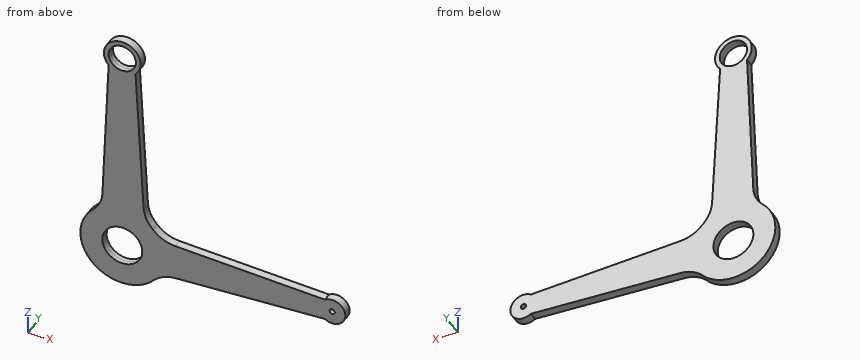
```python
from build123d import *

# Parameters (mm, degrees)
F0_R        = 19.0457812865
F0_R_2      = 13
F0_R_3      = 2.5
F1_DEPTH    = 4
F2_R        = 30
F3_R        = 30
F4_T1_DEPTH = 8
F5_R        = 30


# Not quite as in the source:
# - a fillet or chamfer that OpenCascade refuses, or shapes differently, is made with other operations: its cross-section is extruded or revolved along the edge and cut away or added


with BuildPart() as f1:
    # F0 (on Front) → F1 (new body, symmetric)
    with BuildSketch(Plane.XZ):
        with BuildLine():
            ThreePointArc((-19.5365896508, 34.9044648264), (0.8487956626, 39.99099331), (21, 34.0440890611))
            Line((21, 34.0440890611), (12.6265428967, 187.8830525924))
            ThreePointArc((12.6265428967, 187.8830525924), (-0.2904480488, 182.5024104537), (-13.0217419566, 188.3087966224))
            Line((-13.0217419566, 188.3087966224), (-19.5365896508, 34.9044648264))
        make_face()
        with BuildLine():
            ThreePointArc((35.8133699363, 17.8157945038), (38.939278354, 9.1505519655), (40, 0))
            ThreePointArc((40, 0), (38.9395050251, -9.1495873352), (35.8142525798, -17.8140201007))
            Line((35.8142525798, -17.8140201007), (192.9463185859, -10.3196694961))
            ThreePointArc((192.9463185859, -10.3196694961), (187.5000024995, 0.0079048318), (192.9593762653, 10.3285825468))
            Line((192.9593762653, 10.3285825468), (35.8133699363, 17.8157945038))
        make_face()
        with BuildLine():
            ThreePointArc((35.8142525798, -17.8140201007), (38.9395050251, -9.1495873352), (40, 0))
            ThreePointArc((40, 0), (38.939278354, 9.1505519655), (35.8133699363, 17.8157945038))
            ThreePointArc((35.8133699363, 17.8157945038), (29.542835628, 26.9670328931), (21, 34.0440890611))
            ThreePointArc((21, 34.0440890611), (0.8487956626, 39.99099331), (-19.5365896508, 34.9044648264))
            ThreePointArc((-19.5365896508, 34.9044648264), (-27.5871390481, -28.9646294494), (35.8142525798, -17.8140201007))
        make_face()
        Circle(F0_R, mode=Mode.SUBTRACT)
        with BuildLine():
            ThreePointArc((-13.0217419566, 188.3087966224), (-0.2904480488, 182.5024104537), (12.6265428967, 187.8830525924))
            ThreePointArc((12.6265428967, 187.8830525924), (16.2359862757, 193.4698583741), (17.5, 200))
            ThreePointArc((17.5, 200), (-6.2597729895, 216.3421308929), (-13.0217419566, 188.3087966224))
        make_face()
        with Locations((0, 200)):
            Circle(F0_R_2, mode=Mode.SUBTRACT)
        with BuildLine():
            ThreePointArc((212.5, 0), (205.841327046, 11.0511944306), (192.9593762653, 10.3285825468))
            ThreePointArc((192.9593762653, 10.3285825468), (187.5000024995, 0.0079048318), (192.9463185859, -10.3196694961))
            ThreePointArc((192.9463185859, -10.3196694961), (205.8343372513, -11.0548861974), (212.5, 0))
        make_face()
        with Locations((200, 0)):
            Circle(F0_R_3, mode=Mode.SUBTRACT)
    extrude(amount=F1_DEPTH, both=True)

    # F2
    f2_edges = [f1.edges().sort_by_distance(p)[0] for p in [
        (35.81337, 0, 17.815795),
    ]]
    fillet(f2_edges, radius=F2_R)

    # F3
    f3_edges = [f1.edges().sort_by_distance(p)[0] for p in [
        (21, 0, 34.044089),
    ]]
    fillet(f3_edges, radius=F3_R)

    # F4: fillet of radius 30 on 1 edges, made by hand

    # F4_s2 → F4_t1 (join)
    with BuildSketch(Plane.XZ.offset(-4)):
        with BuildLine():
            ThreePointArc((-18.9466482885, 48.7957428331), (-21.5235892515, 37.8433937284), (-27.954075006, 28.6106569403))
            ThreePointArc((-27.954075006, 28.6106569403), (-23.9529499606, 32.0352335435), (-19.5365896508, 34.9044648264))
            Line((-19.5365896508, 34.9044648264), (-18.9466482885, 48.7957428331))
        make_face()
    extrude(amount=F4_T1_DEPTH)

    # F5
    f5_edges = [f1.edges().sort_by_distance(p)[0] for p in [
        (35.814253, 0, -17.81402),
    ]]
    fillet(f5_edges, radius=F5_R)


solid = f1.part
```
Part model, mm, in its own coordinate system. Give positions to 0.01 mm unless a question says otherwise; leave off trailing zeros. Order: outer loops, then holes, each group sorted by start corner. A loop starts at its lowest first (then second) coordinate and runs counter-clockwise, first axis right, second up. Notation, with made-up numbers: (-13.5, -12.5) - (23.5, -12.5) arc R27 cw to (23.5, 11.5) - close; hole circle Ø11 at (18, 84). An arc over 180 degrees is marked (long way). Use one line per item in the form item = value.
Item 1: Slice it at A-A on y = 2.75. Give the cut face in (x, z).
Solution:
outline = (-27.95, 28.61) arc R40 ccw (long way) to (29.6, -26.91) arc R30 cw to (50.37, -17.12) - (192.95, -10.32) arc R12.5 ccw (long way) to (192.96, 10.33) - (50.37, 17.12) arc R30 cw to (29.6, 26.91) arc R40 ccw to (28.71, 27.85) arc R30 cw to (20.29, 47.11) - (12.63, 187.88) arc R17.5 ccw (long way) to (-13.02, 188.31) - (-18.95, 48.8) arc R30 cw to start; hole circle Ø38.09 at (0, 0); hole circle Ø26 at (0, 200); hole circle Ø5 at (200, 0)
Item 2: Slice it at C-C on z = 200. Give the cut face in (x, y).
Solution:
outline = (-17.5, -4) - (-13, -4) - (-13, 4) - (-17.5, 4) - close; (13, -4) - (17.5, -4) - (17.5, 4) - (13, 4) - close
Item 3: Slice it at B-B on x = 0. Give the cut face in (y, z), and give its area (3 significant figures).
Solution:
outline = (-4, -40) - (4, -40) - (4, -19.05) - (-4, -19.05) - close; (-4, 19.05) - (4, 19.05) - (4, 187) - (-4, 187) - close; (-4, 213) - (4, 213) - (4, 217.5) - (-4, 217.5) - close
area = 1,550 mm2
Item 4: Probe probe 1 along Z at (x, y) = (-12, -0.5); probe 2 along Z at (x, y) = (200, 2.2); probe 3 along X at (y, z) = (3, 47.5). List the from-to ranges inside material, lowest first. Write a range as from..to.
Solution:
probe_1 = -38.16..-14.79, 14.79..195, 205..212.74
probe_2 = -12.5..-2.5, 2.5..12.5
probe_3 = -19.03..20.27
Item 5: Pin check, flat tips, straight feed: pin 1 Ø4 at (x, z) = (200, 0) entering from +Y; pin 2 Ø2 at (y, z) = (0, 34) entering from -X; pin 3 Ø1.5 at (y, z) = (1, 4.5) entering from +X; pin 4 Ø4 at (x, y) = (177.5, -1) entering from -Z. Stop position of each tip, or through.
Solution:
pin_1 = through
pin_2 = -24.25
pin_3 = 211.92
pin_4 = -11.15
Item 6: Slice it at D-D on z = 67. Give the cut face in (x, y), and give its area (3 significant figures).
Solution:
outline = (-18.17, -4) - (19.21, -4) - (19.21, 4) - (-18.17, 4) - close
area = 299 mm2
